```python
from build123d import *

# Parameters (mm, degrees)
BOX016_W     = 12
BOX016_H     = 2
BOX016_DEPTH = 7
BOX018_W     = 3.5
BOX018_H     = 4.3
BOX018_DEPTH = 7
BOX017_W     = 3.5
BOX017_H     = 18
BOX017_DEPTH = 7
BOX015_W     = 2.5
BOX015_H     = 18
BOX015_DEPTH = 7


with BuildPart() as box016:
    # Box016 → Box016 (new body)
    with BuildSketch(Plane(origin=(-9, 17, 0), x_dir=(1, 0, 0), z_dir=(0, 0, 1))):
        with Locations((6, 1)):
            Rectangle(BOX016_W, BOX016_H)
    extrude(amount=BOX016_DEPTH)


with BuildPart() as box018:
    # Box018 → Box018 (new body)
    with BuildSketch(Plane(origin=(-11, 30, 0), x_dir=(1, 0, 0), z_dir=(0, 0, 1))):
        with Locations((1.75, 2.15)):
            Rectangle(BOX018_W, BOX018_H)
    extrude(amount=BOX018_DEPTH)


with BuildPart() as cut043:
    # Box017 → Box017 (new body)
    with BuildSketch(Plane(origin=(-9, 17, 0), x_dir=(1, 0, 0), z_dir=(0, 0, 1))):
        with Locations((1.75, 9)):
            Rectangle(BOX017_W, BOX017_H)
    extrude(amount=BOX017_DEPTH)

    # Cut043: cut Box018
    add(box018.part, mode=Mode.SUBTRACT)


with BuildPart() as fusion020:
    # Box015 → Box015 (new body)
    with BuildSketch(Plane(origin=(1, 1, 0), x_dir=(1, 0, 0), z_dir=(0, 0, 1))):
        with Locations((1.25, 9)):
            Rectangle(BOX015_W, BOX015_H)
    extrude(amount=BOX015_DEPTH)

    # Fusion020: union Box016, Cut043
    add(box016.part)
    add(cut043.part)


solid = fusion020.part
```
Work out the finished part from the listing and answer in its coordinate system (mm). A direction names the side the tool comes from. Coordinates: 2 decimals unless noted, no trailing zeros. Loops run counter-clockwise (first coordinate to the right, second up) from the corner with the lowest first, then second, coordinate; pieces in that order, holes last. Notation, with made-up numbers: M 81,-24 L 139,-24 A14 ccw 139,-19 Z; hole C 46.25,55 d8. An arc over 180 degrees is marked long. Use CSV: the item, a comma, the result in double quotes. Start each with the question number.
(1) Given pin 1 Ø2 at (x, z) = (-3.5, 3) entering from -Y; pin 2 Ø3.5 at (x, z) = (-0.5, 2.5) entering from +Y; pin 3 Ø1 at (y, z) = (22, 4.5) entering from +X, each flat-ended and moving along its own axis, determine where each tip first touches the part or whether it passes through.
(2) Find section B-B, the plane x = -1.5. Give the vertices of the cut face in (y, z), then the cut area to 3 significant figures.
(3) For faces 1 (the face through (-5.5, 27, 3)), 2 (the face through (-9, 23, 3)), 3 (the face through (-4, 17, 3)), 4 (the face through (-3, 18, 0)), 5 (the face through (-8, 34.3, 3)), determine the directions among +Z, -Z, +X, -X, +Y, -Y from which every point of the face is accessible in a straight line to the end or side of a thin tool.
(4) Consider line 1 (X direction, y = 16, z = 1.5); line 2 (X direction, y = 28, z = 1); line 3 (Y direction, x = 2.75, z = 6.5). Determine where each line is inside the solid, lowest interval first.
(5) Find section A-A, the plane z = 6. Give the vertices of the cut face in (x, y).
(6) For a pull along Y with two mould halves and no side action, classify faces 6 (the face through (-1, 19, 3)), 7 (the face through (2, 1, 3)), 8 (the face through (-8, 30, 3)) as +Y half, -Y half, draft (parallel to the pull), parting line (faces both ways), or undercut.
(7) Find section C-C, the plane y = 12. Give the vertices of the cut face in (x, z), then the cut area to 3 significant figures.
Recorded:
1,pin 1,"stops at y = 17"
1,pin 2,"stops at y = 19"
1,pin 3,"stops at x = -5.5"
2,outline,"M 17,0 L 19,0 L 19,7 L 17,7 Z"
2,area,"14.0 mm^2"
3,face 1,"+Z, -Z, +X, +Y"
3,face 2,"+Z, -Z, -X, +Y, -Y"
3,face 3,"+Z, -Z, -X, -Y"
3,face 4,"-Z, +X, -X, +Y, -Y"
3,face 5,"+Z, -Z, -X"
4,line 1,"x = 1 to 3.5"
4,line 2,"x = -9 to -5.5"
4,line 3,"y = 1 to 19"
5,outline,"M -9,17 L 1,17 L 1,1 L 3.5,1 L 3.5,19 L -5.5,19 L -5.5,35 L -9,35 L -9,34.3 L -7.5,34.3 L -7.5,30 L -9,30 Z"
6,face 6,"+Y half"
6,face 7,"-Y half"
6,face 8,"undercut"
7,outline,"M 1,0 L 3.5,0 L 3.5,7 L 1,7 Z"
7,area,"17.5 mm^2"
